from build123d import *

# Parameters (mm, degrees)
ESBO_O1_R                  = 10.35
RESSALTO_EXTRUS_O1_DEPTH   = 2.55
ESBO_O2_R                  = 4.36
ESBO_O2_R_2                = 2.9
RESSALTO_EXTRUS_O2_DEPTH   = 3.1
RESSALTO_EXTRUS_O3_START   = 0.49
ESBO_O3_R                  = 4.36
RESSALTO_EXTRUS_O3_DEPTH   = 0.49
CHANFRO1_SIZE              = 0.48
ESBO_O4_R                  = 3.5
CORTE_EXTRUS_O1_DEPTH      = 1.2
CORTE_EXTRUS_O2_DEPTH      = 7
CORTE_EXTRUS_O2_DEPTH_BACK = 7.2
ESBO_O5_R                  = 1.25
FILETE1_R                  = 0.3
CORTE_EXTRUS_O3_DEPTH      = 2
CORTE_EXTRUS_O3_DEPTH_BACK = 4.2
ESBO_O6_R                  = 0.9
CORTE_EXTRUS_O4_START      = -3.45
ESBO_O8_R                  = 2.9
CORTE_EXTRUS_O4_DEPTH      = 3.45


with BuildPart() as part:
    # Esboço1 → Ressalto-extrusão1 (new body)
    with BuildSketch(Plane.XY):
        Circle(ESBO_O1_R)
    extrude(amount=RESSALTO_EXTRUS_O1_DEPTH)

    # Esboço2 → Ressalto-extrusão2 (add)
    with BuildSketch(Plane.XY.offset(2.55)):
        with Locations(Location((0, 0, 0), (0, 0, 180))):
            Circle(ESBO_O2_R)
        with Locations(Location((0, 0, 0), (0, 0, 180))):
            Circle(ESBO_O2_R_2, mode=Mode.SUBTRACT)
    extrude(amount=RESSALTO_EXTRUS_O2_DEPTH)

    # Esboço3 → Ressalto-extrusão3 (add)
    with BuildSketch(Plane(origin=(0, 0, 0), x_dir=(-1, 0, 0), z_dir=(0, 0, -1)).offset(RESSALTO_EXTRUS_O3_START)):
        Circle(ESBO_O3_R)
    extrude(amount=-RESSALTO_EXTRUS_O3_DEPTH)

    # Chanfro1
    chanfro1_edges = [part.edges().sort_by_distance(p)[0] for p in [
        (4.36, 0, -0.49),
    ]]
    chamfer(chanfro1_edges, length=CHANFRO1_SIZE)

    # Esboço4 → Corte-extrusão1 (cut)
    with BuildSketch(Plane(origin=(0, 0, -0.49), x_dir=(-1, 0, 0), z_dir=(0, 0, -1))):
        Circle(ESBO_O4_R)
    extrude(amount=-CORTE_EXTRUS_O1_DEPTH, mode=Mode.SUBTRACT)

    # Esboço5 → Corte-extrusão2 (cut, two sides: drawn at the far end of the back side and taken through both)
    with BuildSketch(Plane.XY.offset(2.55).offset(-CORTE_EXTRUS_O2_DEPTH_BACK)):
        with Locations(Location((0, 0, 0), (0, 0, 180))):
            Circle(ESBO_O5_R)
    extrude(amount=CORTE_EXTRUS_O2_DEPTH + CORTE_EXTRUS_O2_DEPTH_BACK, mode=Mode.SUBTRACT)

    # Filete1
    filete1_edges = [part.edges().sort_by_distance(p)[0] for p in [
        (4.36, 0, 5.65),
    ]]
    fillet(filete1_edges, radius=FILETE1_R)

    # Esboço6 → Corte-extrusão3 (cut, two sides: drawn at the far end of the back side and taken through both)
    with BuildSketch(Plane.XY.offset(2.55).offset(-CORTE_EXTRUS_O3_DEPTH_BACK)):
        with Locations((0, 7.5)):
            Circle(ESBO_O6_R)
        with Locations((-3.5, 7.5)):
            Circle(ESBO_O6_R)
        with Locations((3.5, 7.5)):
            Circle(ESBO_O6_R)
        with Locations((7.5, 0)):
            Circle(ESBO_O6_R)
        with Locations((7.5, 3.5)):
            Circle(ESBO_O6_R)
        with Locations((7.5, -3.5)):
            Circle(ESBO_O6_R)
        with Locations((-7.5, -3.5)):
            Circle(ESBO_O6_R)
        with Locations((-7.5, 3.5)):
            Circle(ESBO_O6_R)
        with Locations((-7.5, 0)):
            Circle(ESBO_O6_R)
        with Locations((3.5, -7.5)):
            Circle(ESBO_O6_R)
        with Locations((-3.5, -7.5)):
            Circle(ESBO_O6_R)
        with Locations((0, -7.5)):
            Circle(ESBO_O6_R)
    extrude(amount=CORTE_EXTRUS_O3_DEPTH + CORTE_EXTRUS_O3_DEPTH_BACK, mode=Mode.SUBTRACT)

    # Esboço8 → Corte-extrusão4 (cut)
    with BuildSketch(Plane.XY.offset(5.65).offset(CORTE_EXTRUS_O4_START)):
        with Locations(Location((0, 0, 0), (0, 0, 180))):
            Circle(ESBO_O8_R)
    extrude(amount=CORTE_EXTRUS_O4_DEPTH, mode=Mode.SUBTRACT)


solid = part.part
The model under review builds one solid part; all positions refer to its coordinate system, in mm. A direction names the side the tool comes from. Round coordinates to 2 decimals unless told otherwise and drop trailing zeros. Loops run counter-clockwise (first coordinate to the right, second up) from the corner with the lowest first, then second, coordinate; pieces in that order, holes last. Notation, with made-up numbers: M 49,39.25 L 84,39.25 A23 cw 84,71.25 Z; hole C 33,32 d10. An arc over 180 degrees is marked long. Answer as CSV lines item,"result".
1. Insertion check: pin 1 Ø1.5 at (x, z) = (2, 1.5) entering from -Y; pin 2 Ø3 at (x, y) = (0, 0) entering from +Z; pin 3 Ø2.5 at (x, y) = (-7.5, -3.5) entering from -Z. Each pin has a flat end and moves straight along its axis. Give the tip position at first contact, or say it passes through.
Outcome:
pin 1,"stops at y = -10.27"
pin 2,"stops at z = 2.2"
pin 3,"stops at z = 0"
2. We need section B-B (y = 7.25). Give the boundary of the cut face in (x, z).
Outcome:
outline,"M -7.39,0 L -4.36,0 L -4.36,2.55 L -7.39,2.55 Z; M -2.64,0 L -0.86,0 L -0.86,2.55 L -2.64,2.55 Z; M 0.86,0 L 2.64,0 L 2.64,2.55 L 0.86,2.55 Z; M 4.36,0 L 7.39,0 L 7.39,2.55 L 4.36,2.55 Z"
3. We need section A-A (z = 1). Count the separate pieces of the cut face and the enclosed holes in it, plus the area to 3 significant figures.
Outcome:
separate pieces,"1"
enclosed holes,"13"
area,"301 mm2"
4. For faces 1 (the face through (4.5, -2.2, 2.55)), 2 (the face through (-3.233, -1.341, 0.102)), 3 (the face through (1, -3, 5.65)), list the 3-axis set-ups (+Z, -Z, +X, -X, +Y, -Y) from which the entire face can be reached by the end or side of a thin tool; tool diameter is ignored.
Outcome:
face 1,"+Z"
face 2,"-Z"
face 3,"+Z, +X, -X, +Y, -Y"
5. We need section D-D (z = 5). Give the boundary of the cut face in (x, y).
Outcome:
outline,"C 0,0 d8.72; hole C 0,0 d5.8"
6. Draft analysis for pull direction Y (two halves, no side actions). For faces 4 (the face through (4.5, -2.2, 0)), 5 (the face through (-7.695, -4.379, 1.257)), 6 (the face through (0.568, -4.323, 3.93)), state which applies: pulls with the +Y half, pulls with the -Y half, needs draft (parallel to the pull), parting line crosses it, or undercut.
Outcome:
face 4,"needs draft"
face 5,"undercut"
face 6,"parting line crosses it"
7. To check wall thickness, follow L1, parallel to Y at x = 0, z = 1.75; L2, parallel to Y at x = -7.5, z = 1.9. State the ranges of each line that lie inside material, in increasing order. Write a range as [from, to].
Outcome:
L1,"y = [-10.35, -8.4], [-6.6, -1.25], [1.25, 6.6], [8.4, 10.35]"
L2,"y = [-7.13, -4.4], [-2.6, -0.9], [0.9, 2.6], [4.4, 7.13]"
